from build123d import *

# Parameters (mm, degrees)
F0_W     = 7
F0_H     = 1.5
F2_R     = 0.5
F3_DEPTH = 10
F5_DEPTH = 3


with BuildPart() as f1:
    # F0 (on Top) → F1 (revolve)
    with BuildSketch(Plane.XY):
        Polygon((0, 1.5), (0, 0), (3, 0), (3, 1.5), (3, 2.5), (0, 2.5), align=None)
        with Locations((6.5, 0.75)):
            Rectangle(F0_W, F0_H)
    revolve(axis=Axis((5, 0, 0), (1, 0, 0)))

    # F2 (on face) → F3 (cut)
    with BuildSketch(Plane.YZ.offset(10)):
        Circle(F2_R)
    extrude(amount=-F3_DEPTH, mode=Mode.SUBTRACT)

    # F4 (on face) → F5 (cut)
    with BuildSketch(Plane(origin=(0, 0, 0), x_dir=(0, -1, 0), z_dir=(-1, 0, 0))):
        with BuildLine():
            ThreePointArc((0.4974937186, 2.45), (0, 2.5), (-0.4974937186, 2.45))
            ThreePointArc((-0.4974937186, 2.45), (0, 2), (0.4974937186, 2.45))
        make_face()
    extrude(amount=-F5_DEPTH, mode=Mode.SUBTRACT)


solid = f1.part
Could you check a few things on this model? Use its own coordinates, in mm. A direction names the side the tool comes from. Coordinates: 2 decimals unless noted, no trailing zeros. Write each loop counter-clockwise with the first axis right and the second up, starting at its lowest first coordinate (ties: lowest second). Pieces come first, ordered by that corner, then holes. Notation, with made-up numbers: (57.5, -40) - (105.5, -40) arc R25 ccw to (105.5, -9) - close; hole circle Ø7 at (-10.5, -39). An arc over 180 degrees is marked (long way). Put each result on its own line as item: value. Start each with the question number.
Q1. Thinking about a two-plate mould opening in Y: for faces 1 (the cylindrical face through (1, 0, 2)), 2 (the cylindrical face through (1.5, -0.1, -2.5)), 3 (the flat face through (0, 1, 0)), which applies, pulls with the +Y half, pulls with the -Y half, needs draft (parallel to the pull), parting line crosses it, or undercut?
Q2. I want a section at C-C on x = 6.75. Write out the boundary of the cut face in (y, z).
Q3. I want a section at D-D on z = -0.75. Write out the boundary of the cut face in (x, y).
Q4. Which directions (+Z, -Z, +X, -X, +Y, -Y) give clear straight access to the entire face, cutting with the end or side of a thin tool? Please do faces 4 (the flat face through (10, -1, 0)), 5 (the cylindrical face through (6.55, -1.5, 0.07)).
Q5. I want a section at B-B on z = 0. Write out the boundary of the cut face in (x, y).
Q6. Please list where these lines run through material, in increasing order: L1, parallel to Z at x = 6.75, y = 0; L2, parallel to X at y = -1.5, z = -1.2; L3, parallel to Y at x = 1.5, z = 0.2.
Q7. I'm going to push a flat-ended pin straight in: P1, Ø3, axis at x = 6, y = 1, coming from the +Z side. Where does the tip first touch, or does it pass through?
Q8. I want a section at A-A on y = 0. Write out the boundary of the cut face in (x, z), plus the area to 3 significant figures.
Checks:
1. face 1: undercut
1. face 2: parting line crosses it
1. face 3: needs draft
2. outline: circle Ø3 at (0, 0); hole circle Ø1 at (0, 0)
3. outline: (0, -2.38) - (3, -2.38) - (3, -1.3) - (10, -1.3) - (10, 1.3) - (3, 1.3) - (3, 2.38) - (0, 2.38) - close
4. face 4: +Z, -Z, +X, +Y, -Y
4. face 5: +X
5. outline: (0, -2.5) - (3, -2.5) - (3, -1.5) - (10, -1.5) - (10, -0.5) - (0, -0.5) - close; (0, 0.5) - (10, 0.5) - (10, 1.5) - (3, 1.5) - (3, 2.5) - (0, 2.5) - close
6. L1: -1.5 to -0.5, 0.5 to 1.5
6. L2: 0 to 3
6. L3: -2.49 to -0.46, 0.46 to 2.49
7. P1: z = 1.5
8. outline: (0, -2.5) - (3, -2.5) - (3, -1.5) - (10, -1.5) - (10, -0.5) - (0, -0.5) - close; (0, 0.5) - (10, 0.5) - (10, 1.5) - (3, 1.5) - (3, 2) - (0, 2) - close
8. area: 24.5 mm²
